Part model, mm, in its own coordinate system. Face numbers are marked on the shaded views. A direction names the side the tool comes from. Give positions to 0.01 mm unless a question says otherwise; leave off trailing zeros. Write each loop counter-clockwise with the first axis right and the second up, starting at its lowest first coordinate (ties: lowest second). Pieces come first, ordered by that corner, then holes. Notation, with made-up numbers: M -27,74.25 L 31,74.25 A26 cw 31,107.25 Z; hole C 29,21.5 d9. An arc over 180 degrees is marked long. Write item = value, one per line. Start each with the question number.
from build123d import *

# Parameters (mm, degrees)
SKETCH1_W                        = 254
SKETCH1_H                        = 254
BOSS_EXTRUDE1_DEPTH              = 9.525
SKETCH2_W                        = 25.4
SKETCH2_H                        = 50.8
CUT_EXTRUDE1_DEPTH               = 180.857514786
SKETCH4_W                        = 53.975
SKETCH4_H                        = 50.8
CUT_EXTRUDE2_DEPTH               = 4.7625
SKETCH7_W                        = 9.525
SKETCH7_H                        = 38.1
CUT_EXTRUDE4_DEPTH               = 180.857514786
F_10_0_1935_DIAMETER_HOLE1_D     = 4.9149
F_10_0_1935_DIAMETER_HOLE1_DEPTH = 12.7
F_10_0_1935_DIAMETER_HOLE1_TIP   = 1.476584928
F_10_0_1935_DIAMETER_HOLE3_D     = 4.9149
F_10_0_1935_DIAMETER_HOLE3_DEPTH = 12.7
F_10_0_1935_DIAMETER_HOLE3_TIP   = 1.476584928
SKETCH16_R                       = 0.79375
CUT_EXTRUDE7_DEPTH               = 180.668253752
SKETCH17_W                       = 254
SKETCH17_H                       = 101.6
CUT_EXTRUDE8_DEPTH               = 180.857514786


with BuildPart() as part:
    # Sketch1 → Boss-Extrude1 (new body)
    with BuildSketch(Plane(origin=(0, 0, 0), x_dir=(1, 0, 0), z_dir=(0, 1, 0))):
        Rectangle(SKETCH1_W, SKETCH1_H)
    extrude(amount=BOSS_EXTRUDE1_DEPTH)

    # Sketch2 → Cut-Extrude1 (cut, through all)
    with BuildSketch(Plane(origin=(0, 9.525, 0), x_dir=(1, 0, 0), z_dir=(0, 1, 0))):
        with Locations((-114.3, 101.6)):
            Rectangle(SKETCH2_W, SKETCH2_H)
        with Locations((114.3, 101.6)):
            Rectangle(SKETCH2_W, SKETCH2_H)
    extrude(amount=-CUT_EXTRUDE1_DEPTH, mode=Mode.SUBTRACT)

    # Sketch4 → Cut-Extrude2 (cut)
    with BuildSketch(Plane(origin=(0, 9.525, 0), x_dir=(1, 0, 0), z_dir=(0, 1, 0))):
        with Locations((-74.6125, 101.6)):
            Rectangle(SKETCH4_W, SKETCH4_H)
        with Locations((74.6125, 101.6)):
            Rectangle(SKETCH4_W, SKETCH4_H)
    extrude(amount=-CUT_EXTRUDE2_DEPTH, mode=Mode.SUBTRACT)

    # Sketch7 → Cut-Extrude4 (cut, through all)
    with BuildSketch(Plane(origin=(0, 9.525, 0), x_dir=(1, 0, 0), z_dir=(0, 1, 0))):
        with Locations((-122.2375, 25.4)):
            Rectangle(SKETCH7_W, SKETCH7_H)
        with Locations((122.2375, 25.4)):
            Rectangle(SKETCH7_W, SKETCH7_H)
    extrude(amount=-CUT_EXTRUDE4_DEPTH, mode=Mode.SUBTRACT)

    # #10 (0.1935) Diameter Hole1
    with Locations(Plane(origin=(117.475, 0, 0), x_dir=(0, 0, -1), z_dir=(1, 0, 0))):
        with Locations((11.1125, 4.7625), (39.6875, 4.7625)):
            Hole(F_10_0_1935_DIAMETER_HOLE1_D / 2, depth=F_10_0_1935_DIAMETER_HOLE1_DEPTH)
            with Locations((0, 0, -(F_10_0_1935_DIAMETER_HOLE1_DEPTH + F_10_0_1935_DIAMETER_HOLE1_TIP / 2))):  # 118° drill point
                Cone(0, F_10_0_1935_DIAMETER_HOLE1_D / 2, F_10_0_1935_DIAMETER_HOLE1_TIP, mode=Mode.SUBTRACT)

    # #10 (0.1935) Diameter Hole3
    with Locations(Plane.ZY.offset(117.475)):
        with Locations((-39.6875, 4.7625), (-11.1125, 4.7625)):
            Hole(F_10_0_1935_DIAMETER_HOLE3_D / 2, depth=F_10_0_1935_DIAMETER_HOLE3_DEPTH)
            with Locations((0, 0, -(F_10_0_1935_DIAMETER_HOLE3_DEPTH + F_10_0_1935_DIAMETER_HOLE3_TIP / 2))):  # 118° drill point
                Cone(0, F_10_0_1935_DIAMETER_HOLE3_D / 2, F_10_0_1935_DIAMETER_HOLE3_TIP, mode=Mode.SUBTRACT)

    # Sketch16 → Cut-Extrude7 (cut, through all)
    with BuildSketch(Plane(origin=(0, 4.7625, 0), x_dir=(1, 0, 0), z_dir=(0, 1, 0))):
        with Locations(Location((93.599, 117.221, 0), (0, 0, 270))):
            Circle(SKETCH16_R)
        with Locations(Location((55.499, 117.221, 0), (0, 0, 270))):
            Circle(SKETCH16_R)
        with Locations(Location((55.499, 85.979, 0), (0, 0, 270))):
            Circle(SKETCH16_R)
        with Locations(Location((93.599, 85.979, 0), (0, 0, 270))):
            Circle(SKETCH16_R)
        with Locations(Location((-93.599, 85.979, 0), (0, 0, 270))):
            Circle(SKETCH16_R)
        with Locations(Location((-55.499, 85.979, 0), (0, 0, 270))):
            Circle(SKETCH16_R)
        with Locations(Location((-55.499, 117.221, 0), (0, 0, 270))):
            Circle(SKETCH16_R)
        with Locations(Location((-93.599, 117.221, 0), (0, 0, 270))):
            Circle(SKETCH16_R)
    extrude(amount=-CUT_EXTRUDE7_DEPTH, mode=Mode.SUBTRACT)

    # Sketch17 → Cut-Extrude8 (cut, through all)
    with BuildSketch(Plane(origin=(0, 9.525, 0), x_dir=(1, 0, 0), z_dir=(0, 1, 0))):
        with Locations((0, -76.2)):
            Rectangle(SKETCH17_W, SKETCH17_H)
    extrude(amount=-CUT_EXTRUDE8_DEPTH, mode=Mode.SUBTRACT)


solid = part.part
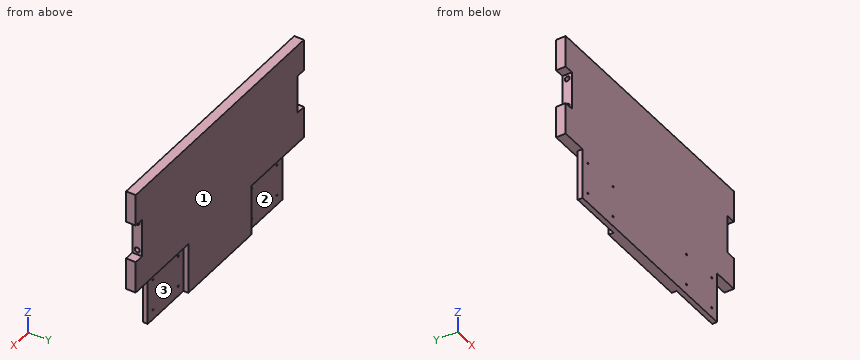
Q1. Slice it at B-B (x = -77). Give the cut face in (y, z) (1 decimal).
Q2. Probe line 1 along X through (y, z) = (0.5, -113); line 2 along Z through (x, y) = (112, 2); line 3 along X through (y, z) = (8.5, -98.5) (3 decimals). List the from-to ranges inside material, lowest first.
Q3. Tool access for the marked faces 1, 2 and 3: list every direction of +Z, -Z, +X, -X, +Y, -Y with a clear straight run to the whole face (end or side of a thin tool).
Q4. Drop flat-ended pins along their axis: P1, Ø6, axis at x = 4, z = -104, coming from the -Y side; P2, Ø5, axis at x = 121, y = 3.5, coming from the -Z side; P3, Ø5.5, axis at y = 4.76, z = -39.69, coming from the -X side (3 decimals); P4, Ø1.4, axis at y = 8, z = -111.5, coming from the +X side (3 decimals). Give the stop position or say it passes through.
Q5. Slice it at A-A (z = -94). Give the cut face in (x, y) (1 decimal), and give its area (3 significant figures).
Working result:
q1.outline = M 0,-127 L 4.8,-127 L 4.8,-76.2 L 9.5,-76.2 L 9.5,25.4 L 0,25.4 Z
q2.line_1 = -101.6 to 101.6
q2.line_2 = -76.2 to 25.4
q2.line_3 = -47.625 to 47.625
q3.face_1 = +Z, -Z, +X, -X, +Y
q3.face_2 = -Z, -X, +Y
q3.face_3 = -Z, +X, +Y
q4.P1 = 0
q4.P2 = -76.2
q4.P3 = -117.475
q4.P4 = 47.625
q5.outline = M -101.6,0 L 101.6,0 L 101.6,4.8 L 47.6,4.8 L 47.6,9.5 L -47.6,9.5 L -47.6,4.8 L -101.6,4.8 Z
q5.area = 1,420 mm2
